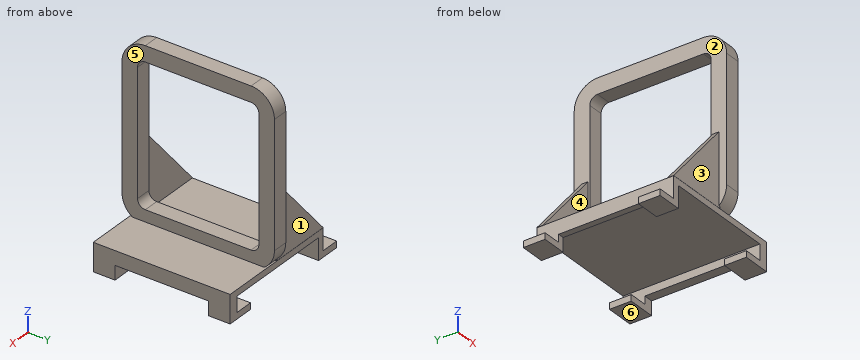
```python
from build123d import *

# Parameters (mm, degrees)
F1_DEPTH = 22
F2_W     = 2
F2_H     = 2.5
F2_W_2   = 3
F4_DEPTH = 15
F6_W     = 5
F6_H     = 5
F9_DEPTH = 2


with BuildPart() as f1:
    # F0 (on Front) → F1 (new body)
    with BuildSketch(Plane.XZ):
        Polygon((-22.3971781656, 0), (-28.3971781656, 0), (-28.3971781656, -2), (-20.3971781656, -2), (-20.3971781656, 5), (13.6028218344, 5), (15.6028218344, 5), (15.6028218344, 0), (9.6028218344, 0), (9.6028218344, -2), (18.6028218344, -2), (18.6028218344, 7), (-22.3971781656, 7), align=None)
    extrude(amount=F1_DEPTH)

    # F2 (on face) → F4 (cut)
    with BuildSketch(Plane.XZ.offset(22)):
        Polygon((-20.3971781656, 0), (-22.3971781656, 0), (-28.3971781656, 0), (-28.3971781656, -2), (-20.3971781656, -2), align=None)
        Polygon((18.6028218344, -2), (18.6028218344, 0), (15.6028218344, 0), (9.6028218344, 0), (9.6028218344, -2), align=None)
        with Locations((-21.3971781656, 1.25)):
            Rectangle(F2_W, F2_H)
        with Locations((17.1028218344, 1.25)):
            Rectangle(F2_W_2, F2_H)
    extrude(amount=-F4_DEPTH, mode=Mode.SUBTRACT)

    # F7: sweep along a path in F3
    with BuildLine(Plane.YZ) as f7_path:
        Line((-22.250123322, 8.247365728), (-5, 8.247365728))
        ThreePointArc((-5, 8.247365728), (-1.4644660941, 9.7118318221), (0, 13.247365728))
        Line((0, 13.247365728), (0, 53.247365728))
        ThreePointArc((0, 53.247365728), (-1.4644660941, 56.782899634), (-5, 58.247365728))
        Line((-5, 58.247365728), (-22.250123322, 58.247365728))
    # F6 (on offset) → F7 (sweep)
    with BuildSketch(Plane.XZ.offset(22)):
        with Locations((0, 8.247365728)):
            Rectangle(F6_W, F6_H)
    sweep(path=f7_path.line)

    # F8 (on Front) → F9 (join)
    with BuildSketch(Plane.XZ):
        Polygon((-1.9540686626, 30.8402627707), (-22.409658879, 7.0511708036), (-1.9540686626, 7.0511708036), align=None)
    extrude(amount=F9_DEPTH)

    # F10: F1 across plane


with BuildPart() as f1_1:
    add(f1.part)
    add(f1.part.mirror(Plane.XZ.offset(22)))


solid = f1_1.part
```
Geometry: final body of the model. Coordinates: model frame, mm. Face numbers are marked on the shaded views. A direction names the side the tool comes from. Round coordinates to 2 decimals unless told otherwise and drop trailing zeros. Order: outer loops, then holes, each group sorted by start corner. A loop starts at its lowest first (then second) coordinate and runs counter-clockwise, first axis right, second up. Notation, with made-up numbers: (79, -9.5) - (113, -9.5) arc R20 cw to (113, -3.5) - close; hole circle Ø3 at (6, -11.75). An arc over 180 degrees is marked (long way). Write item = value, one per line. Start each with the question number.
Q1. Ray query, line 1 (Y direction, x = 0, z = 31); line 2 (Y direction, x = -3.5, z = 9.5); line 3 (Y direction, x = -4.5, z = 5.5). Return the intervals inside material, ascending. Write a range as from..to.
Q2. Access query for the marked faces 4, 5 and 6. Directions: +Z, -Z, +X, -X, +Y, -Y. A direction counts if a zero-diameter tool reaches every point of the face in a straight line with its end or side. Return the directions, or none.
Q3. Pin query (flat end, axial travel): pin 1 (6 mm diameter, centred on x = -8.5, z = 20.5, fed in from -Y); pin 2 (7 mm diameter, centred on x = -1.5, z = 4.5, fed in from -Y); pin 3 (8 mm diameter, centred on y = -28, z = 14, fed in from -X); pin 4 (12 mm diameter, centred on x = -12.5, z = 49, fed in from +Y). Return the tip coordinate at first contact, or that it passes through.
Q4. Cut plane C-C on y = -29. Return the cut outline in (x, z).
Q5. Cut plane A-A on z = 4. Return the cut outline in (x, y).
Q6. Cut plane D-D on x = -5.5. Return the cut outline in (y, z).
Q7. Cut plane B-B on x = -23.5. Return the cut outline in (y, z), and give its area (3 significant figures).
Q8. Pull-direction query (Y, two-part tool) for the marked faces 1, 2 and 3; classes: +Y half, -Y half, draft (parallel to the pull), parting line (faces both ways), or undercut.
Outcome:
q1.line_1 = -46.5..-41.5, -2.5..2.5
q1.line_2 = -44..-42, -2..0
q1.line_3 = -44..0
q2.face_4 = +Z, -X
q2.face_5 = +Z, +X, +Y, -Y
q2.face_6 = -Z, +X, -X, +Y, -Y
q3.pin_1 = -44
q3.pin_2 = -44.36
q3.pin_3 = -2.5
q3.pin_4 = through
q4.outline = (-22.4, 2.5) - (-20.4, 2.5) - (-20.4, 5) - (15.6, 5) - (15.6, 2.5) - (18.6, 2.5) - (18.6, 7) - (2.5, 7) - (2.5, 10.75) - (-2.5, 10.75) - (-2.5, 7) - (-22.4, 7) - close; (-2.5, 55.75) - (2.5, 55.75) - (2.5, 60.75) - (-2.5, 60.75) - close
q5.outline = (-22.4, -44) - (-20.4, -44) - (-20.4, 0) - (-22.4, 0) - close; (15.6, -44) - (18.6, -44) - (18.6, 0) - (15.6, 0) - close
q6.outline = (-44, 5) - (0, 5) - (0, 7) - (-44, 7) - close; (-44, 7.05) - (-42, 7.05) - (-42, 26.72) - (-44, 26.72) - close; (-2, 7.05) - (0, 7.05) - (0, 26.72) - (-2, 26.72) - close
q7.outline = (-44, -2) - (-37, -2) - (-37, 0) - (-44, 0) - close; (-7, -2) - (0, -2) - (0, 0) - (-7, 0) - close
q7.area = 28.0 mm^2
q8.face_1 = +Y half
q8.face_2 = undercut
q8.face_3 = -Y half
